Can you work these out from the drawing? Everything is in mm from the part's minimum corner. A direction names the side the tool comes from. Give positions to 0.01 mm unless a question says otherwise; leave off trailing zeros. Loops run counter-clockwise (first coordinate to the right, second up) from the corner with the lowest first, then second, coordinate; pieces in that order, holes last.
Q1. For the marked faces 1 and 2, which set-ups out of +Z, -Z, +X, -X, +Y, -Y let a thin tool reach every point of the face, with its end or its side?
Q2. If we section it at A-A (z = 8): Please give me the cut outline in (x, y).
Q3. If we section it at B-B (y = 3.25): Please give me the cut outline in (x, z), plus the area to 3 significant figures.
Q4. Will these pins go through, and if not, where does the flat tip stop? P1, Ø2.5, axis at y = 5, z = 7.5, coming from the -X side; P2, Ø1, axis at x = 8, z = 3.5, coming from the +Y side; P3, Ø1.5, axis at x = 29.5, y = 4, coming from the +Z side.
Q5. If we section it at D-D (z = 4): Please give me the cut outline in (x, y) (1 decimal), plus the area to 3 significant figures.
Q6. If we section it at C-C (x = 30.5): Please give me the cut outline in (y, z).
Q7. I need wall thicknesses on line 1 (X direction, y = 3.75, z = 8.75); line 2 (X direction, y = 2.25, z = 7) (1 decimal); line 3 (Y direction, x = 36.5, z = 1.25). Which ranges of each line are inside material? Lowest first, please.
Q8. We'd pull the mould along X, two halves only. Please class the marked faces 3, 4, 5 and 6: +X half, -X half, draft (parallel to the pull), parting line (faces both ways), or undercut.
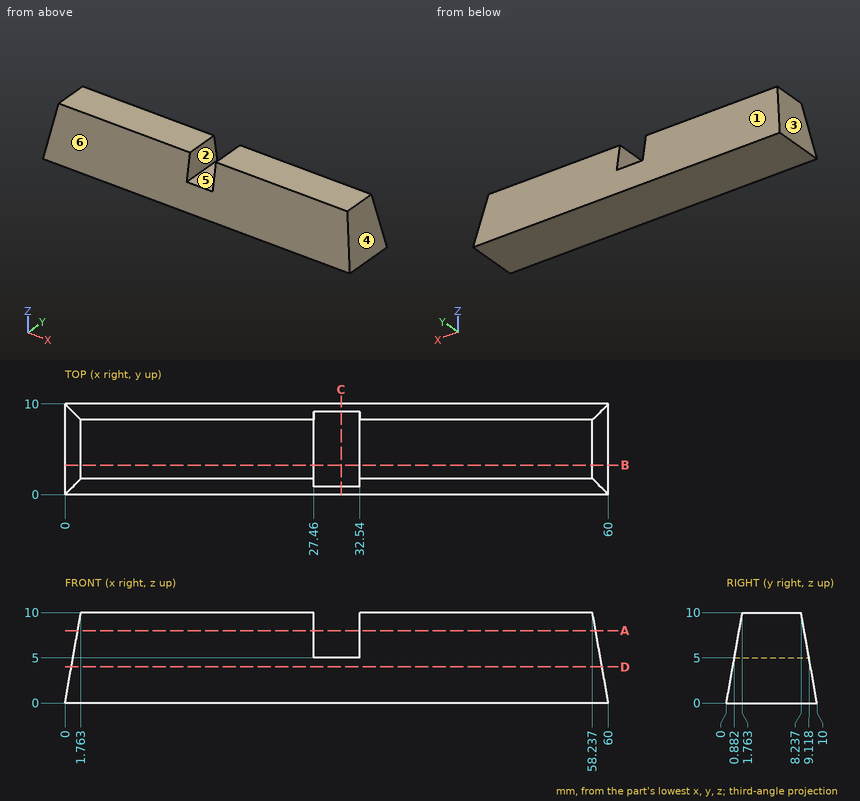
Check sheet entries:
1. face 1: +Z, +X, -X, +Y
1. face 2: +Z, +Y, -Y
2. outline: (1.41, 1.41) - (27.46, 1.41) - (27.46, 8.59) - (1.41, 8.59) - close; (32.54, 1.41) - (58.59, 1.41) - (58.59, 8.59) - (32.54, 8.59) - close
3. outline: (0, 0) - (60, 0) - (58.24, 10) - (32.54, 10) - (32.54, 5) - (27.46, 5) - (27.46, 10) - (1.76, 10) - close
3. area: 557 mm2
4. P1: stops at x = 1.1
4. P2: stops at y = 9.47
4. P3: stops at z = 5
5. outline: (0.7, 0.7) - (59.3, 0.7) - (59.3, 9.3) - (0.7, 9.3) - close
5. area: 503 mm2
6. outline: (0, 0) - (10, 0) - (9.12, 5) - (0.88, 5) - close
7. line 1: x = 1.54 to 27.46, 32.54 to 58.46
7. line 2: x = 1.2 to 27.5, 32.5 to 58.8
7. line 3: y = 0.22 to 9.78
8. face 3: -X half
8. face 4: +X half
8. face 5: undercut
8. face 6: draft
